Source: CAD feature listing. Evaluate the final solid. Frame: model axes, mm. Face numbers are marked on the shaded views. A direction names the side the tool comes from. Round coordinates to 2 decimals unless told otherwise and drop trailing zeros. Answer in a Markdown table with one row per item. Add a question column.
```python
from build123d import *

# Parameters (mm, degrees)
SKETCH_R        = 7
PAD_DEPTH       = 15
CHAMFER_SIZE    = 2
SKETCH003_W     = 150
SKETCH003_H     = 8
POCKET001_DEPTH = 0.75
POCKET002_DEPTH = 15.001
POCKET003_DEPTH = 15.001
CHAMFER002_SIZE = 2


with BuildPart() as part:
    # Sketch → Pad (new body)
    with BuildSketch(Plane.YZ):
        with BuildLine():
            Line((0, 10), (0, 55.1837281655))
            ThreePointArc((11.9080899538, 65), (3.6392177972, 62.8999739994), (0, 55.1837281655))
            Line((11.9080899538, 65), (166.5070947684, 34.9489976518))
            ThreePointArc((166.5070947684, 34.9489976518), (168.0070985661, 35.2541768735), (168.851967126, 36.5306340279))
            Line((169.4243941122, 39.4755155782), (168.851967126, 36.5306340279))
            ThreePointArc((171.7345605988, 41.063580806), (170.2546752416, 40.7420394634), (169.4243941122, 39.4755155782))
            ThreePointArc((180, 31.2151647136), (177.6598174256, 37.6437879725), (171.7345605988, 41.063580806))
            Line((180, 31.2151647136), (180, 10))
            ThreePointArc((170, 0), (177.0710678119, 2.9289321881), (180, 10))
            Line((170, 0), (10, 0))
            ThreePointArc((0, 10), (2.9289321881, 2.9289321881), (10, 0))
        make_face()
        with Locations((16, 16)):
            Circle(SKETCH_R, mode=Mode.SUBTRACT)
    extrude(amount=PAD_DEPTH)

    # Chamfer
    chamfer_edges = [part.edges().sort_by_distance(p)[0] for p in [
        (15, 90, 0),
        (0, 90, 0),
    ]]
    chamfer(chamfer_edges, length=CHAMFER_SIZE)

    # Sketch003 (on Face1 of Pad) → Pocket001 (cut)
    with BuildSketch(Plane.YX):
        with Locations((90, 7.5)):
            Rectangle(SKETCH003_W, SKETCH003_H)
    extrude(amount=-POCKET001_DEPTH, mode=Mode.SUBTRACT)

    # Sketch004 (on Face14 of Pad) → Pocket002 (cut, through all)
    with BuildSketch(Plane.YZ.offset(15)):
        with BuildLine():
            Line((21.8351520655, 37.4576612912), (47.3574588351, 32.4966274114))
            ThreePointArc((47.3574588351, 32.4966274114), (58.6177903834, 38.7723375448), (54.336603861, 50.9317391014))
            ThreePointArc((51.9639954797, 56.1952040061), (52.3138370776, 53.1864198979), (54.336603861, 50.9317391014))
            Line((51.9639954797, 56.1952040061), (52.1548044751, 57.1768311896))
            Line((52.1548044751, 57.1768311896), (26.6324977055, 62.1378650694))
            Line((26.6324977055, 62.1378650694), (26.4416887101, 61.1562378859))
            ThreePointArc((22.2701158683, 57.1648329504), (24.9902108638, 58.4975948081), (26.4416887101, 61.1562378859))
            ThreePointArc((22.2701158683, 57.1648329504), (13.7456768513, 47.4945928448), (21.8351520655, 37.4576612912))
        make_face()
        with BuildLine():
            Line((121.463034607, 18.091962684), (146.9853413767, 13.1309288042))
            ThreePointArc((146.9853413767, 13.1309288042), (158.2456729249, 19.4066389377), (153.9644864025, 31.5660404943))
            ThreePointArc((151.5918780213, 36.829505399), (151.9417196191, 33.8207212907), (153.9644864025, 31.5660404943))
            Line((151.5918780213, 36.829505399), (151.7826870167, 37.8111325824))
            Line((151.7826870167, 37.8111325824), (126.260380247, 42.7721664622))
            Line((126.260380247, 42.7721664622), (126.0695712516, 41.7905392787))
            ThreePointArc((121.8979984099, 37.7991343433), (124.6180934053, 39.1318962009), (126.0695712516, 41.7905392787))
            ThreePointArc((121.8979984099, 37.7991343433), (113.3735593928, 28.1288942377), (121.463034607, 18.091962684))
        make_face()
    extrude(amount=-POCKET002_DEPTH, mode=Mode.SUBTRACT)

    # Sketch005 (on Face14 of Pad) → Pocket003 (cut, through all)
    with BuildSketch(Plane.YZ.offset(15)):
        with BuildLine():
            Line((90.3363821208, 9), (40, 9))
            ThreePointArc((35, 14), (36.4644660941, 10.4644660941), (40, 9))
            Line((35, 14), (35, 23.8844015175))
            ThreePointArc((40.9540449769, 28.7925374348), (36.8196088986, 27.7425244345), (35, 23.8844015175))
            Line((40.9540449769, 28.7925374348), (91.2904270977, 19.0081359172))
            ThreePointArc((95.3363821208, 14.1), (94.1945050377, 17.2803911014), (91.2904270977, 19.0081359172))
            Line((95.3363821208, 14.1), (95.3363821208, 14))
            ThreePointArc((90.3363821208, 9), (93.8719160267, 10.4644660941), (95.3363821208, 14))
        make_face()
    extrude(amount=-POCKET003_DEPTH, mode=Mode.SUBTRACT)

    # Chamfer002
    chamfer002_edges = [part.edges().sort_by_distance(p)[0] for p in [
        (15, 66.122236, 23.900337),
        (0, 66.122236, 23.900337),
    ]]
    chamfer(chamfer002_edges, length=CHAMFER002_SIZE)


solid = part.part
```
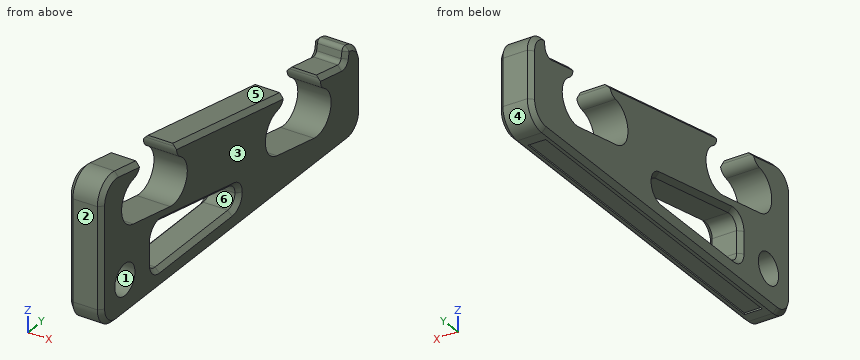
(1) Draft query along Y for the marked faces 1, 2, 3 and 4. Return one class per face: +Y half, -Y half, draft (parallel to the pull), parting line (faces both ways), or undercut.
(2) Line query: line 1 (Z direction, x = 4.75, y = 16); line 2 (Y direction, x = 10, z = 38.5); line 3 (Z direction, x = 12.75, y = 47). Output: solid intervals per line, ascending. Write a range as from..to.
(3) Access query for the marked faces 5 and 6. Directions: +Z, -Z, +X, -X, +Y, -Y. A direction counts if a zero-diameter tool reaches every point of the face in a straight line with its end or side. Return the directions, or none.
(4) Cut plane A-A (x = 6). Count the separate pieces of the cut face and the enclosed holes in it, and give its area (3 significant figures).
(5) Pin query (flat end, axial travel): pin 1 (1 mm diameter, centred on x = 11, y = 153, fed in from +Z); pin 2 (1 mm diameter, centred on x = 11, z = 42.5, fed in from +Y); pin 3 (12.5 mm diameter, centred on y = 16, z = 16, fed in from -X); pin 4 (2.5 mm diameter, centred on x = 6, y = 62.5, fed in from -Z). Return the tip coordinate at first contact, or that it passes through.
Answer list:
| question | item | result |
|---|---|---|
| 1 | face 1 | undercut |
| 1 | face 2 | -Y half |
| 1 | face 3 | draft |
| 1 | face 4 | +Y half |
| 2 | line 1 | 0.75..9, 23..40.95, 53.6..64.2 |
| 2 | line 2 | 0..18.95, 58.51..123.8, 169.23..176.85 |
| 2 | line 3 | 0..9, 27.62..32.57 |
| 3 | face 5 | +Z, +X, -X, +Y |
| 3 | face 6 | +X, -X |
| 4 | separate pieces | 1 |
| 4 | enclosed holes | 2 |
| 4 | area | 5,850 mm² |
| 5 | pin 1 | z = 37.67 |
| 5 | pin 2 | y = 126.26 |
| 5 | pin 3 | through |
| 5 | pin 4 | z = 0.75 |
